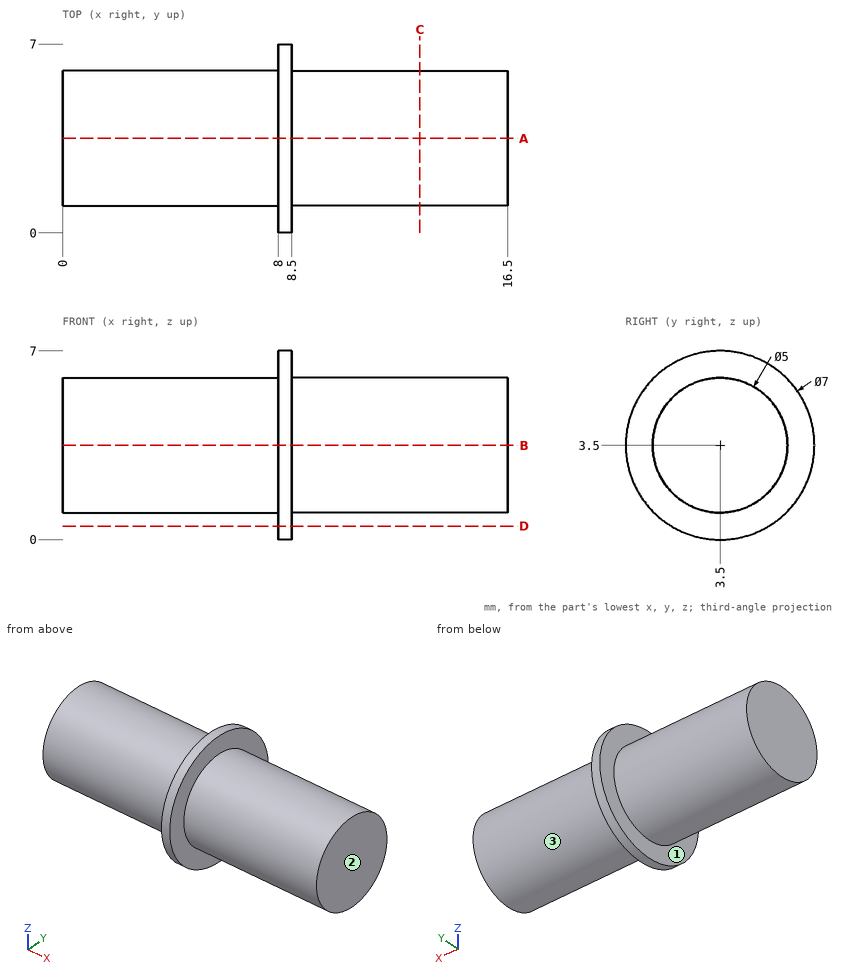
Study the drawing (mm; zero at the part's minimum x, y, z) and answer. A direction names the side the tool comes from. Round coordinates to 2 decimals unless told otherwise and drop trailing zeros. Write each loop counter-clockwise with the first axis right and the second up, starting at its lowest first coordinate (ties: lowest second). Pieces come first, ordered by that corner, then holes. Notation, with made-up numbers: (59.25, 73) -> (80.25, 73) arc R19 cw to (80.25, 107) -> close; hole circle Ø7 at (68, 6). An arc over 180 degrees is marked (long way). Use CSV: the item, a comma, the result in double quotes. Start each with the question number.
(1) Consider L1, parallel to X at y = 6, z = 1.25; L2, parallel to Z at x = 2, y = 4.5; L3, parallel to Z at x = 13.5, y = 3.75. Determine where each line is inside the solid, lowest interval first. Write a range as from..to.
(2) Section A-A on y = 3.5 is taken. Give the vertices of the cut face in (x, z), then the cut area to 3 significant figures.
(3) Each of these flat-tipped pins is pushed along its axis until it touches: pin 1 (4 mm diameter, centred on x = 4, y = 5.5, fed in from -Z); pin 2 (1.5 mm diameter, centred on x = 5.5, y = 1, fed in from -Z); pin 3 (1 mm diameter, centred on x = 7, y = 5.5, fed in from -Z). Where does it stop, or does it pass through?
(4) Section C-C on x = 13.25 is taken. Give the vertices of the cut face in (y, z).
(5) Section D-D on z = 0.5 is taken. Give the vertices of the cut face in (x, y).
(6) Which of the six approach directions +Z, -Z, +X, -X, +Y, -Y give full straight-line access (tool end or side, diameter ignored) to the marked faces 1, 2 and 3?
A:
1,L1,"x = 8..8.5"
1,L2,"z = 1.21..5.79"
1,L3,"z = 1.01..5.99"
2,outline,"(0, 1) -> (8, 1) -> (8, 0) -> (8.5, 0) -> (8.5, 1) -> (16.5, 1) -> (16.5, 6) -> (8.5, 6) -> (8.5, 7) -> (8, 7) -> (8, 6) -> (0, 6) -> close"
2,area,"83.5 mm²"
3,pin 1,"stops at z = 1"
3,pin 2,"stops at z = 1.71"
3,pin 3,"stops at z = 1.5"
4,outline,"circle Ø5 at (3.5, 3.5)"
5,outline,"(8, 1.7) -> (8.5, 1.7) -> (8.5, 5.3) -> (8, 5.3) -> close"
6,face 1,"-X"
6,face 2,"+Z, -Z, +X, +Y, -Y"
6,face 3,"+X"
